from build123d import *

# Parameters (mm, degrees)
SKETCH_1_W          = 40
SKETCH_1_H          = 30
SKETCH_1_W_2        = 38
SKETCH_1_H_2        = 28
EXTRUDE_1_DEPTH     = 100
SKETCH_2_R          = 1.6
CUT_EXTRUDE_1_DEPTH = 112.803398875
SKETCH_3_R          = 1.6
CUT_EXTRUDE_2_DEPTH = 112.803398875
SKETCH_4_R          = 1.6
CUT_EXTRUDE_3_DEPTH = 112.803398875


with BuildPart() as part:
    # 草图1 → 拉伸-薄壁1 (new body)
    with BuildSketch(Plane(origin=(0, 0, 0), x_dir=(1, 0, 0), z_dir=(0, 1, 0))):
        with Locations((20, 15)):
            Rectangle(SKETCH_1_W, SKETCH_1_H)
        with Locations((20, 15)):
            Rectangle(SKETCH_1_W_2, SKETCH_1_H_2, mode=Mode.SUBTRACT)
    extrude(amount=EXTRUDE_1_DEPTH)

    # 草图2 → 切除-拉伸1 (cut, through all)
    with BuildSketch(Plane.XY):
        with Locations((5, 95)):
            Circle(SKETCH_2_R)
        with Locations((35, 95)):
            Circle(SKETCH_2_R)
        with Locations((35, 25)):
            Circle(SKETCH_2_R)
        with Locations((5, 25)):
            Circle(SKETCH_2_R)
        with Locations((5, 5)):
            Circle(SKETCH_2_R)
        with Locations((35, 5)):
            Circle(SKETCH_2_R)
    extrude(amount=-CUT_EXTRUDE_1_DEPTH, mode=Mode.SUBTRACT)

    # 草图3 → 切除-拉伸2 (cut, through all)
    with BuildSketch(Plane.ZY):
        with Locations((-25, 90)):
            Circle(SKETCH_3_R)
        with Locations((-5, 90)):
            Circle(SKETCH_3_R)
        with Locations((-25, 10)):
            Circle(SKETCH_3_R)
        with Locations((-5, 10)):
            Circle(SKETCH_3_R)
    extrude(amount=-CUT_EXTRUDE_2_DEPTH, mode=Mode.SUBTRACT)

    # 草图4 → 切除-拉伸3 (cut, through all)
    with BuildSketch(Plane.XY):
        with Locations((16, 67)):
            Circle(SKETCH_4_R)
    extrude(amount=-CUT_EXTRUDE_3_DEPTH, mode=Mode.SUBTRACT)


solid = part.part
Can you work these out from the model? Positions are in its coordinate system, mm. A direction names the side the tool comes from. Round coordinates to 2 decimals unless told otherwise and drop trailing zeros. Write each loop counter-clockwise with the first axis right and the second up, starting at its lowest first coordinate (ties: lowest second). Pieces come first, ordered by that corner, then holes. Notation, with made-up numbers: (70, 49.25) -> (109, 49.25) arc R23 cw to (109, 76.25) -> close; hole circle Ø9 at (6.5, -35.75). An arc over 180 degrees is marked (long way). Use one line per item in the form item = value. Start each with the question number.
Q1. I'm going to push a flat-ended pin straight in: P1, Ø3, axis at y = 10, z = -25, coming from the +X side. Where does the tip first touch, or does it pass through?
Q2. Imagine slicing it at A-A (z = -5). Please give me the cut outline in (x, y).
Q3. Which directions (+Z, -Z, +X, -X, +Y, -Y) give clear straight access to the entire face, cutting with the end or side of a thin tool? Please do faces 4 (the face through (20, 49, -29)), 5 (the face through (18.4, 100, -0.6)).
Q4. We'd pull the mould along X, two halves only. Please class faces 1 (the face through (1, 49, -15)), 2 (the face through (0.493, 91.586, -25.208)), 3 (the face through (0, 49, -15)): +X half, -X half, draft (parallel to the pull), parting line (faces both ways), or undercut.
Q5. Imagine slicing it at C-C (x = 30). Please give me the cut outline in (y, z), then the cut area to 3 significant figures.
Q6. Imagine slicing it at D-D (y = 34). Please give me the cut outline in (x, z), then the cut area to 3 significant figures.
Q7. Imagine slicing it at B-B (y = 67). Please give me the cut outline in (x, z).
Q8. If I drill on probe 1 along Y at (x, z) = (5, -0.4); probe 2 along X at (y, z) = (95, -29.5); probe 3 along Y at (x, z) = (0.5, -5), over which ranges is the centre line in solid material (lowest first)? Write a range as [from, to].
Worked out:
q1.P1 = through
q2.outline = (0, 0) -> (1, 0) -> (1, 8.4) -> (0, 8.4) -> close; (0, 11.6) -> (1, 11.6) -> (1, 88.4) -> (0, 88.4) -> close; (0, 91.6) -> (1, 91.6) -> (1, 100) -> (0, 100) -> close; (39, 0) -> (40, 0) -> (40, 8.4) -> (39, 8.4) -> close; (39, 11.6) -> (40, 11.6) -> (40, 88.4) -> (39, 88.4) -> close; (39, 91.6) -> (40, 91.6) -> (40, 100) -> (39, 100) -> close
q3.face_4 = +Y, -Y
q3.face_5 = +Z, -Z, +X, -X, +Y
q4.face_1 = undercut
q4.face_2 = draft
q4.face_3 = -X half
q5.outline = (0, -30) -> (100, -30) -> (100, -29) -> (0, -29) -> close; (0, -1) -> (100, -1) -> (100, 0) -> (0, 0) -> close
q5.area = 200 mm^2
q6.outline = (0, -30) -> (40, -30) -> (40, 0) -> (0, 0) -> close; hole (1, -29) -> (39, -29) -> (39, -1) -> (1, -1) -> close
q6.area = 136 mm^2
q7.outline = (0, -30) -> (14.4, -30) -> (14.4, -29) -> (1, -29) -> (1, -1) -> (14.4, -1) -> (14.4, 0) -> (0, 0) -> close; (17.6, -30) -> (40, -30) -> (40, 0) -> (17.6, 0) -> (17.6, -1) -> (39, -1) -> (39, -29) -> (17.6, -29) -> close
q8.probe_1 = [0, 3.4], [6.6, 23.4], [26.6, 93.4], [96.6, 100]
q8.probe_2 = [0, 3.4], [6.6, 33.4], [36.6, 40]
q8.probe_3 = [0, 8.4], [11.6, 88.4], [91.6, 100]
